from build123d import *

# Parameters (mm, degrees)
BOSS_EXTRUDE1_DEPTH = 10
SKETCH3_W           = 20
SKETCH3_H           = 50
BOSS_EXTRUDE2_DEPTH = 40
CUT_EXTRUDE1_DEPTH  = 40
SKETCH5_W           = 50
SKETCH5_H           = 20
BOSS_EXTRUDE3_DEPTH = 30
CUT_EXTRUDE2_DEPTH  = 30


with BuildPart() as part:
    # Sketch2 → Boss-Extrude1 (new body)
    with BuildSketch(Plane(origin=(0, 0, 0), x_dir=(1, 0, 0), z_dir=(0, 1, 0))):
        Polygon((0, 50), (0, 10), (60, 10), (60, 0), (80, 0), (80, 50), align=None)
    extrude(amount=BOSS_EXTRUDE1_DEPTH)

    # Sketch3 → Boss-Extrude2 (add)
    with BuildSketch(Plane(origin=(0, 10, 0), x_dir=(1, 0, 0), z_dir=(0, 1, 0))):
        with Locations((70, 25)):
            Rectangle(SKETCH3_W, SKETCH3_H)
    extrude(amount=BOSS_EXTRUDE2_DEPTH)

    # Sketch4 → Cut-Extrude1 (cut)
    with BuildSketch(Plane(origin=(80, 0, 0), x_dir=(0, 0, -1), z_dir=(1, 0, 0))):
        Polygon((20, 50), (0, 30), (0, 50), align=None)
    extrude(amount=-CUT_EXTRUDE1_DEPTH, mode=Mode.SUBTRACT)

    # Sketch5 → Boss-Extrude3 (add)
    with BuildSketch(Plane(origin=(0, 10, 0), x_dir=(1, 0, 0), z_dir=(0, 1, 0))):
        with Locations((35, 40)):
            Rectangle(SKETCH5_W, SKETCH5_H)
    extrude(amount=BOSS_EXTRUDE3_DEPTH)

    # Sketch6 → Cut-Extrude2 (cut)
    with BuildSketch(Plane.XY.offset(-30)):
        Polygon((40, 40), (10, 20), (10, 40), align=None)
    extrude(amount=-CUT_EXTRUDE2_DEPTH, mode=Mode.SUBTRACT)


solid = part.part
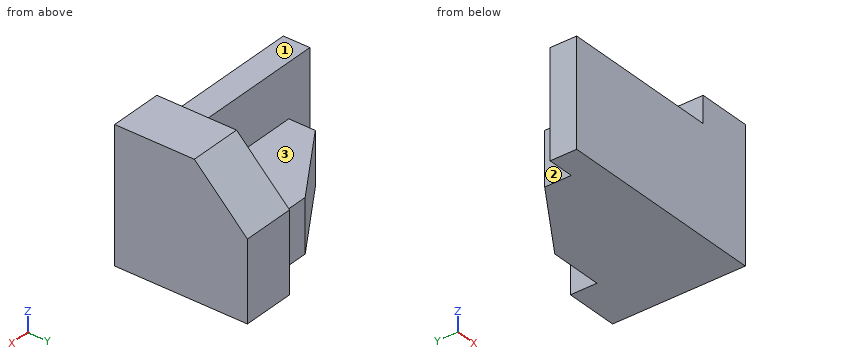
Model file for the job. Use its own axes, mm. Face numbers are marked on the shaded views. A direction names the side the tool comes from. Give positions to 0.01 mm unless a question says otherwise; leave off trailing zeros. Order: outer loops, then holes, each group sorted by start corner. A loop starts at its lowest first (then second) coordinate and runs counter-clockwise, first axis right, second up. Notation, with made-up numbers: (10, 55) -> (14, 55) arc R22 ccw to (14, 77) -> close; hole circle Ø7 at (-9.75, 29.5). An arc over 180 degrees is marked (long way). Use CSV: the item, a comma, the result in double quotes.
1. 3-axis set-ups, long thin cutter, end or side, ignore diameter. For the marked faces 1, 2 and 3: which of +Z, -Z, +X, -X, +Y, -Y reach the whole face in a straight line?
Outcome:
face 1,"+Z, -X, +Y, -Y"
face 2,"+Z, -Z, -X, +Y"
face 3,"+Z, -X, +Y"
2. Drop flat-ended pins along their axis: pin 1 (11 mm diameter, centred on x = 26.5, y = 3.5, fed in from +Z); pin 2 (5 mm diameter, centred on y = 13.5, z = -35, fed in from -X); pin 3 (15 mm diameter, centred on x = 46, y = 21.5, fed in from +Z). Give the stop position or say it passes through.
Outcome:
pin 1,"z = -10"
pin 2,"x = 10"
pin 3,"z = -30"
3. Drill centre lines: line 1 along Z through (x, y) = (37.5, 20); line 2 along X through (y, z) = (29.5, -25.5); line 3 along X through (y, z) = (18, -47.5). Where is each one in solid material? Low to high. Write a range as from..to.
Outcome:
line 1,"-50..-30"
line 2,"60..80"
line 3,"10..80"
4. Band-saw the part on A-A, the plane z = -39.5. Give the cut face in (x, y), then the cut area to 3 significant figures.
Outcome:
outline,"(0, 0) -> (80, 0) -> (80, 50) -> (60, 50) -> (60, 40) -> (40, 40) -> (10, 20) -> (10, 10) -> (0, 10) -> close"
area,"2,800 mm²"
5. Band-saw the part on C-C, the plane x = 34. Give the cut face in (y, z).
Outcome:
outline,"(0, -50) -> (36, -50) -> (36, -30) -> (10, -30) -> (10, -10) -> (0, -10) -> close"
6. Band-saw the part on B-B, the plane y = 24. Give the cut face in (x, z).
Outcome:
outline,"(16, -50) -> (80, -50) -> (80, 0) -> (60, 0) -> (60, -30) -> (16, -30) -> close"
7. Band-saw the part on D-D, the plane y = 45. Give the cut face in (x, z).
Outcome:
outline,"(60, -50) -> (80, -50) -> (80, -15) -> (60, -15) -> close"
